from build123d import *

# Parameters (mm, degrees)
SKETCH1_R           = 3.5
BOSS_EXTRUDE1_DEPTH = 35
CUT_EXTRUDE1_START  = 10
SKETCH3_R           = 0.75
CUT_EXTRUDE1_DEPTH  = 20
SKETCH4_R           = 6
BOSS_EXTRUDE2_DEPTH = 3


with BuildPart() as part:
    # Sketch1 → Boss-Extrude1 (new body)
    with BuildSketch(Plane.XY):
        Circle(SKETCH1_R)
    extrude(amount=BOSS_EXTRUDE1_DEPTH)

    # Sketch3 → Cut-Extrude1 (cut)
    with BuildSketch(Plane(origin=(0, 0, 0), x_dir=(1, 0, 0), z_dir=(0, 1, 0)).offset(CUT_EXTRUDE1_START)):
        with Locations(Location((0, -8, 0), (0, 0, 270))):
            Circle(SKETCH3_R)
    extrude(amount=-CUT_EXTRUDE1_DEPTH, mode=Mode.SUBTRACT)

    # Sketch4 → Boss-Extrude2 (add)
    with BuildSketch(Plane.XY.offset(35)):
        Circle(SKETCH4_R)
    extrude(amount=BOSS_EXTRUDE2_DEPTH)


solid = part.part
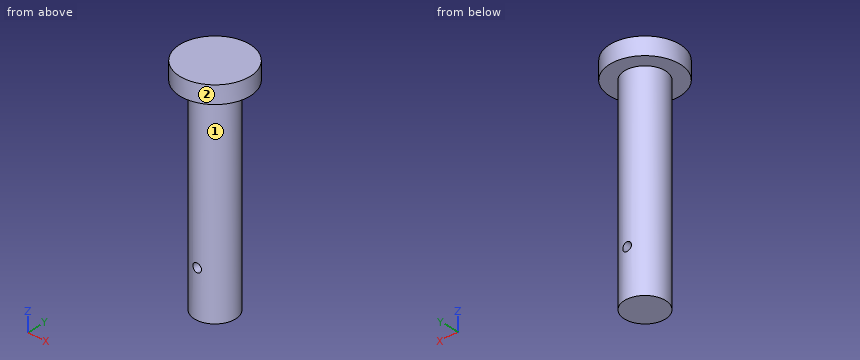
Read the model definition and answer for the solid it produces. Units are mm, in the model's axes. Face numbers are marked on the shaded views. A direction names the side the tool comes from. Round coordinates to 2 decimals unless told otherwise and drop trailing zeros. Write each loop counter-clockwise with the first axis right and the second up, starting at its lowest first coordinate (ties: lowest second). Pieces come first, ordered by that corner, then holes.
1. The part is cut by section D-D, the plane x = -3. Determine the outline of the cut face in (y, z).
2. Straight lines are drawn through the part: L1, parallel to Z at x = 0, y = 2; L2, parallel to X at y = 0.25, z = 8; L3, parallel to Y at x = -0.25, z = 18.5. For each, find the intervals that lie inside material, in ascending order.
3. The part is cut by section A-A, the plane x = 0. Determine the outline of the cut face in (y, z).
4. The part is cut by section C-C, the plane z = 36. Determine the outline of the cut face in (x, y).
5. Given pin 1 Ø1.7 at (x, z) = (0, 8) entering from -Y; pin 2 Ø1.5 at (y, z) = (2.5, 27.5) entering from -X; pin 3 Ø4 at (y, z) = (-2.5, 8.5) entering from -X, each flat-ended and moving along its own axis, determine where each tip first touches the part or whether it passes through.
6. The part is cut by section B-B, the plane y = 0. Determine the outline of the cut face in (x, z).
7. Which of the six approach directions +Z, -Z, +X, -X, +Y, -Y give full straight-line access (tool end or side, diameter ignored) to the marked faces 1 and 2?
Values:
1. outline: (-5.2, 35) - (-1.8, 35) - (-1.8, 0) - (1.8, 0) - (1.8, 35) - (5.2, 35) - (5.2, 38) - (-5.2, 38) - close
2. L1: z = 0 to 7.25, 8.75 to 38
2. L2: x = -3.49 to -0.75, 0.75 to 3.49
2. L3: y = -3.49 to 3.49
3. outline: (-6, 35) - (-3.5, 35) - (-3.5, 8.75) - (3.5, 8.75) - (3.5, 35) - (6, 35) - (6, 38) - (-6, 38) - close; (-3.5, 0) - (3.5, 0) - (3.5, 7.25) - (-3.5, 7.25) - close
4. outline: circle Ø12 at (0, 0)
5. pin 1: stops at y = -3.5
5. pin 2: stops at x = -3.03
5. pin 3: stops at x = -3.46
6. outline: (-6, 35) - (-3.5, 35) - (-3.5, 0) - (3.5, 0) - (3.5, 35) - (6, 35) - (6, 38) - (-6, 38) - close; hole circle Ø1.5 at (0, 8)
7. face 1: -Z
7. face 2: +Z, -Z
